The drawing under review shows one solid part. Ordinate dimensions are in mm from its lowest x, y, z. A direction names the side the tool comes from. Round coordinates to 2 decimals unless told otherwise and drop trailing zeros. Order: outer loops, then holes, each group sorted by start corner. A loop starts at its lowest first (then second) coordinate and runs counter-clockwise, first axis right, second up.
1) To check wall thickness, follow L1, parallel to Y at x = 9.5, z = 19.5; L2, parallel to X at y = 8.75, z = 15.25; L3, parallel to Y at x = 11.75, z = 22.5. State the ranges of each line that lie inside material, in increasing order.
2) Mouldability with a two-part tool opening along X and no side actions: class the marked faces 3, 4 and 5 as pulls with the +X half, pulls with the -X half, needs draft (parallel to the pull), parting line crosses it, or undercut.
3) Clearance check with flat-ended pins moving along their axes: P1, Ø6, axis at y = 15, z = 22, coming from the +X side; P2, Ø1.5, axis at x = 3.5, z = 8.5, coming from the +Y side; P3, Ø4, axis at x = 9.5, y = 9.5, coming from the +Z side. State where each tip first meets the part, or that it passes through.
4) Consider section D-D (z = 18.75). Give the boundary of the cut face in (x, y), then the cut area to 3 significant figures.
5) Machinability: for the marked faces 1 and 2, which of the approach directions +Z, -Z, +X, -X, +Y, -Y give a long, thin tool a straight path to every point of the face, cutting with its end or side? Answer none if there is none.
6) Consider section C-C (z = 7.75). Give the boundary of the cut face in (x, y), then the cut area to 3 significant figures.
7) Consider section A-A (x = 9.5). Give the boundary of the cut face in (y, z).
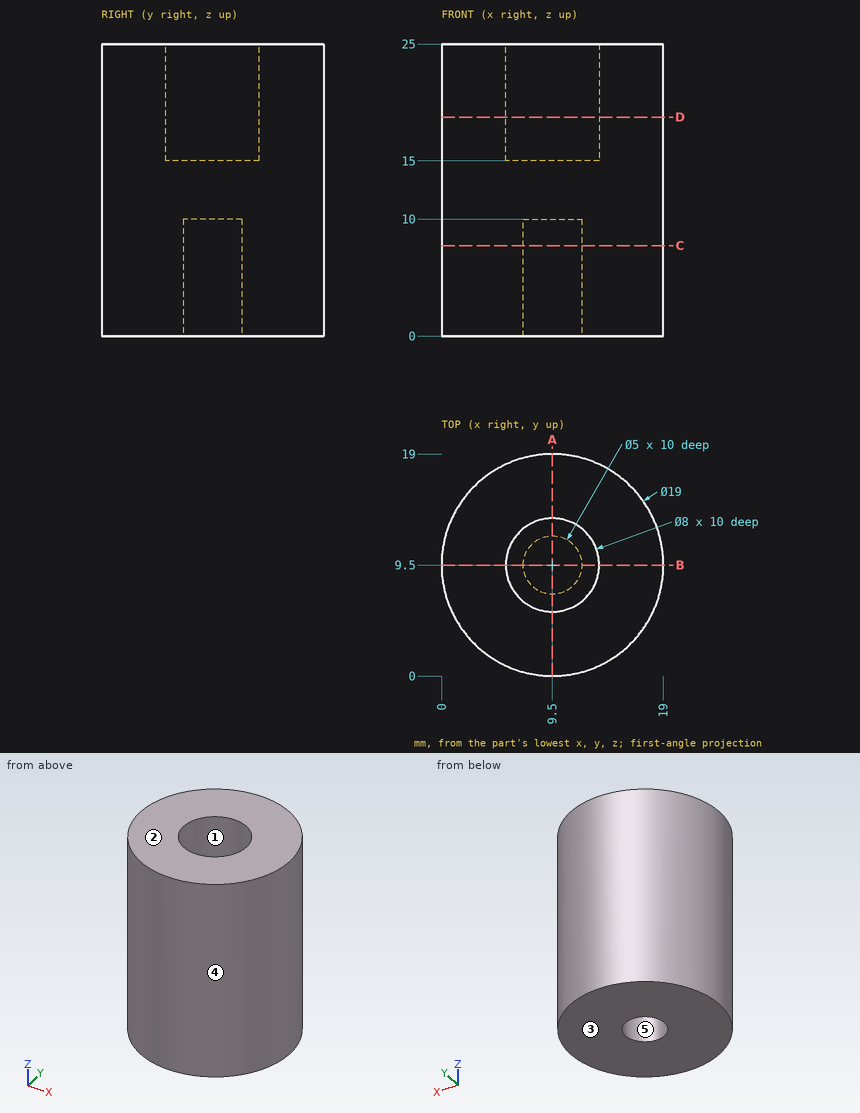
Answer below:
1. L1: y = 0 to 5.5, 13.5 to 19
1. L2: x = 0.03 to 5.57, 13.43 to 18.97
1. L3: y = 0.27 to 6.19, 12.81 to 18.73
2. face 3: needs draft
2. face 4: parting line crosses it
2. face 5: undercut
3. P1: stops at x = 18.67
3. P2: stops at y = 17.42
3. P3: stops at z = 15
4. outline: circle Ø19 at (9.5, 9.5); hole circle Ø8 at (9.5, 9.5)
4. area: 233 mm2
5. face 1: +Z
5. face 2: +Z, +X, -X, +Y, -Y
6. outline: circle Ø19 at (9.5, 9.5); hole circle Ø5 at (9.5, 9.5)
6. area: 264 mm2
7. outline: (0, 0) - (7, 0) - (7, 10) - (12, 10) - (12, 0) - (19, 0) - (19, 25) - (13.5, 25) - (13.5, 15) - (5.5, 15) - (5.5, 25) - (0, 25) - close
